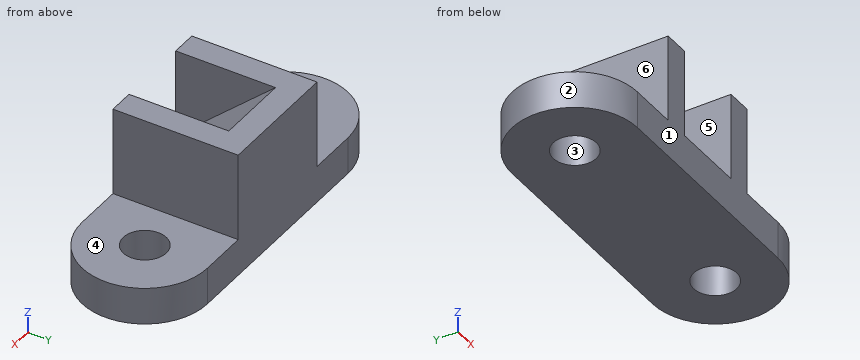
Autodesk Fusion 360 part; units mm, degrees
sketch "base" plane through (0, 0, 0) normal (0, 0, 1) x (1, 0, 0)
  line L0 (-35, -17) -> (79, -17)
  line L1 (79, 47) -> (-35, 47)
  circle A0 centre (-35, 15) radius 11
  circle A1 centre (79, 15) radius 11
  arc A2 (79, -17) -> (79, 47) centre (79, 15) ccw
  arc A3 (-35, 47) -> (-35, -17) centre (-35, 15) ccw
  dimension "d1" = 114
  dimension "d2" = 64
  dimension "d3" = 22
  dimension "d4" = 22
extrude "Extrude1" add sketch "base" along normal blind 19
sketch "middle" plane through (0, 0, 19) normal (0, 0, 1) x (-1, 0, 0)
  circle A0 centre (-79, -15) radius 11
  circle A1 centre (35, -15) radius 11
  arc A2 (35, -47) -> (35, 17) centre (35, -15) ccw
  line L0 (35, 17) -> (-79, 17)
  arc A3 (-79, 17) -> (-79, -47) centre (-79, -15) ccw
  line L1 (-79, -47) -> (35, -47)
  line L2 (-22, -47) -> (-3, -47)
  line L3 (-22, -47) -> (-41, -47)
  line L4 (-22, -47) -> (-54, -47)
  line L5 (-22, -47) -> (10, -47)
  line L6 (10, -47) -> (10, 17)
  line L7 (10, 17) -> (-3.0614, 17)
  line L8 (-3.0614, 17) -> (-3.0614, -34)
  line L9 (-54, -47) -> (-54, 17)
  line L10 (-54, 17) -> (-41, 17)
  line L11 (-41, 17) -> (-41, -34)
  line L12 (-41, -34) -> (-3.0614, -34)
  dimension "d10" = 32
  dimension "d11" = 32
  dimension "d12" = 51
extrude "Extrude2" add sketch "middle" along normal blind 45 contours L0 L8 L11 L12
sketch "ramp" plane through (41, 0, 0) normal (1, 0, 0) x (0, 1, 0)
  line L0 (-17, 19) -> (34, 19)
  line L1 (34, 19) -> (34, 64)
  line L2 (34, 64) -> (-17, 64)
  line L3 (-17, 64) -> (-17, 19)
  line L4 (34, 64) -> (-17, 19)
  line L5 (-17, 64) -> (-17, 19)
  line L6 (-17, 64) -> (34, 64)
extrude "Extrude3" cut sketch "ramp" against normal blind 38 contours L2 L3 L4 L5 L6
extrude "Extrude4" add sketch "middle" along normal blind 45 contours L0 L1 L2 L3 L4 L5 L6 L7 L8 L9 L10 L11 L12
Here's how the part is built. I have some questions about the finished solid (model axes, mm). Face numbers are marked on the shaded views. A direction names the side the tool comes from. Coordinates: 2 decimals unless noted, no trailing zeros. Order: outer loops, then holes, each group sorted by start corner. A loop starts at its lowest first (then second) coordinate and runs counter-clockwise, first axis right, second up. Notation, with made-up numbers: (70.25, 25.5) - (107.25, 25.5) arc R29 ccw to (107.25, 53.5) - close; hole circle Ø8 at (32.25, 81). An arc over 180 degrees is marked (long way). Use CSV: the item, a comma, the result in double quotes. Start each with the question number.
1. For the marked faces 4, 5 and 6, which set-ups out of +Z, -Z, +X, -X, +Y, -Y let a thin tool reach every point of the face, with its end or its side?
2. Please list where these lines run through material, in increasing order: line 1 (Y direction, x = -35, z = 11); line 2 (X direction, y = 10, z = 10); line 3 (X direction, y = -12, z = 55). Write a range as from..to.
3. Suppose I cut it at C-C on x = -27. List the corners of the cut face in (y, z) for me.
4. I'm going to push flat-ended pins straight in: pin 1 (13.5 mm diameter, centred on y = 15.5, z = 40.5, fed in from -X); pin 2 (4 mm diameter, centred on x = 9.5, z = 25, fed in from -Y); pin 3 (5 mm diameter, centred on y = 1, z = 8, fed in from +X); pin 4 (17.5 mm diameter, centred on x = -35, y = 15, fed in from -Z). Where does each tip first touch, or does it pass through?
5. Suppose I cut it at D-D on x = 23. List the corners of the cut face in (y, z) for me.
6. Suppose I cut it at B-B on z = 59.5. List the corners of the cut face in (x, y) for me, then the cut area to 3 significant figures.
7. Suppose I cut it at A-A on y = 24. List the corners of the cut face in (x, z) for me.
8. If we mould it in two halves opening along Y, with no side actions, what happens to the marked faces 1, 2 and 3? For each: +Y half, -Y half, draft (parallel to the pull), parting line (faces both ways), or undercut.
Output:
1,face 4,"+Z, +X, +Y, -Y"
1,face 5,"+Z, -Y"
1,face 6,"+Z, -X, +Y, -Y"
2,line 1,"y = -17..4, 26..47"
2,line 2,"x = -66.61..-44.8, -25.2..69.2, 88.8..110.61"
2,line 3,"x = -10..3.06, 41..54"
3,outline,"(-17, 0) - (7.45, 0) - (7.45, 19) - (-17, 19) - close; (22.55, 0) - (47, 0) - (47, 19) - (22.55, 19) - close"
4,pin 1,"stops at x = -10"
4,pin 2,"stops at y = -12.47"
4,pin 3,"stops at x = 108.86"
4,pin 4,"passes through"
5,outline,"(-17, 0) - (47, 0) - (47, 64) - (34, 64) - (-17, 19) - close"
6,outline,"(-10, -17) - (3.06, -17) - (3.06, 28.9) - (41, 28.9) - (41, -17) - (54, -17) - (54, 47) - (-10, 47) - close"
6,area,"2,350 mm2"
7,outline,"(-65.71, 0) - (-41.32, 0) - (-41.32, 19) - (-65.71, 19) - close; (-28.68, 0) - (72.68, 0) - (72.68, 19) - (54, 19) - (54, 64) - (41, 64) - (41, 55.18) - (3.06, 55.18) - (3.06, 64) - (-10, 64) - (-10, 19) - (-28.68, 19) - close; (85.32, 0) - (109.71, 0) - (109.71, 19) - (85.32, 19) - close"
8,face 1,"-Y half"
8,face 2,"parting line"
8,face 3,"undercut"
